Solid Edge part; units mm, degrees
sketch "Sketch1" plane through (0, 0, 0) normal (0, -1, 0) x (1, 0, 0)
  line L0 (2.5, 0) -> (5, 2.5)
  line L1 (5, 2.5) -> (5, 2.8)
  line L2 (5, 2.8) -> (0, 2.8)
  line L3 (0, 2.8) -> (0, -11.2)
  line L4 (0, -11.2) -> (2.0095, -11.2)
  line L5 (2.0095, -11.2) -> (2.5, -10.7095)
  line L6 (2.5, -10.7095) -> (2.5, -2.4)
  line L7 (2.5, -2.4) -> (2.0095, -2.4)
  line L8 (2.0095, -2.4) -> (2.0095, -2.39)
  line L9 (2.0095, -2.39) -> (2.5, -2.39)
  line L10 (2.5, -2.39) -> (2.5, 0)
  dimension "D1" = 2.5
  dimension "D2" = 2.0095
revolve "RevolvedProtrusion1" add sketch "Sketch1" angle 360 about axis through (0, 0, 54) along (0, 0, -1)
sketch "Sketch2" plane through (0, 0, 0) normal (0, -1, 0) x (1, 0, 0)
  arc A0 (-1.5, 0.5) -> (0, 0) centre (0, 2.5) ccw
  line L0 (0, 0.5) -> (0, 0)
  line L1 (-1.5, 0.5) -> (0, 0.5)
revolve "RevolvedCutout1" cut sketch "Sketch2" angle 360 about axis through (0, 0, 54) along (0, 0, -1)
sketch "Sketch3" plane through (0, 0, 2.8) normal (0, 0, 1) x (0, -1, 0)
  line L0 (-1.7321, 0) -> (-0.866, 1.5)
  line L1 (-0.866, 1.5) -> (0.866, 1.5)
  line L2 (0.866, 1.5) -> (1.7321, 0)
  line L3 (1.7321, 0) -> (0.866, -1.5)
  line L4 (0.866, -1.5) -> (-0.866, -1.5)
  line L5 (-0.866, -1.5) -> (-1.7321, 0)
extrude "Cutout1" cut sketch "Sketch3" against normal blind 2.3
cosmetic_thread "Thread1"
sketch "Sketch4" plane through (0, 0, 0) normal (1, 0, 0) x (0, 1, 0)
  line L0 (-1.72, 2.8) -> (0, 1.807)
revolve "RevolvedCutout2" cut sketch "Sketch4" angle 360 about axis through (0, 0, -57) along (0, 0, 1) material side at (0, -0.835, 2.3468)
fillet "Round1" radius 0.2 1 edges at (-2.5, 0, 0)
properties material "Stahl"
The listing builds one solid part. Answer for the finished solid, in the listing's coordinates (mm). A direction names the side the tool comes from. Round coordinates to 2 decimals unless told otherwise and drop trailing zeros. Write each loop counter-clockwise with the first axis right and the second up, starting at its lowest first coordinate (ties: lowest second). Pieces come first, ordered by that corner, then holes. Notation, with made-up numbers: (-2, 10.5) -> (14, 10.5) arc R24 cw to (14, 42.5) -> close; hole circle Ø6 at (-36.5, 74). An arc over 180 degrees is marked (long way). Answer as a JSON object with one key per item and string values. Group by question number.
Q1. Section B-B (z = -6.75) is taken. Write down the section's boundary in (x, y).
Q2. Straight lines are drawn through the part: line 1 along X through (y, z) = (-2, -8.75); line 2 along Y through (x, z) = (-0.5, 2.25); line 3 along X through (y, z) = (-2, 1.25). For each, find the intervals that lie inside material, in ascending order.
Q3. Section A-A (z = 1) is taken. Write down the section's boundary in (x, y).
Q4. Which of the six approach directions +Z, -Z, +X, -X, +Y, -Y give full straight-line access (tool end or side, diameter ignored) to faces 4 (the face through (1.5, 0, 2)), 5 (the face through (4.77, 1.5, 2.65))?
Q5. Determine the mould class of faces 1 (the face through (2, 0, 2.8)), 2 (the face through (-0.74, -1.305, 1.666)), 3 (the face through (-0.54, -2.44, -6.5)) for opening direction X: pulls with the +X half, pulls with the -X half, needs draft (parallel to the pull), parting line crosses it, or undercut.
Q6. Each of these flat-tipped pins is pushed along its axis until it touches: pin 1 Ø2 at (y, z) = (-1.5, -1.5) entering from -X; pin 2 Ø5 at (x, z) = (2.5, -3) entering from -Y; pin 3 Ø5 at (y, z) = (4, -0.5) entering from +X. Where does it stop, or does it pass through?
Check values:
{
 "1": {"outline": "circle Ø5 at (0, 0)"},
 "2": {"line 1": "-1.5 to 1.5", "line 2": "-4.72 to -1.44, 1.44 to 4.72", "line 3": "-3.17 to 3.17"},
 "3": {"outline": "circle Ø7 at (0, 0); hole (-1.5, -0.87) -> (0, -1.73) -> (1.5, -0.87) -> (1.5, 0.87) -> (0, 1.73) -> (-1.5, 0.87) -> close"},
 "4": {"face 4": "+Z", "face 5": "+Z, -Z"},
 "5": {"face 1": "needs draft", "face 2": "undercut", "face 3": "parting line crosses it"},
 "6": {"pin 1": "x = -2.45", "pin 2": "y = -2.5", "pin 3": "x = 3.13"}
}
